For this review, take the finished solid that the model builds, in its own axes (mm). Face numbers are marked on the shaded views. A direction names the side the tool comes from. Coordinates: 2 decimals unless noted, no trailing zeros. Loops run counter-clockwise (first coordinate to the right, second up) from the corner with the lowest first, then second, coordinate; pieces in that order, holes last. Notation, with made-up numbers: (-14, 44.25) - (-1, 44.25) arc R9 ccw to (-1, 60.25) - close; hole circle Ø6 at (13, 78.25). An arc over 180 degrees is marked (long way). One line per item, written item: value. Start each with the question number.
1. Take a section at D-D, the plane z = -16.5. State the section outline as (x, y) points.
2. Take a section at B-B, the plane y = 4. State the section outline as (x, z) points, and give its area (3 significant figures).
3. For the marked faces 1, 2 and 3, list the 3-axis set-ups (+Z, -Z, +X, -X, +Y, -Y) from which the entire face can be reached by the end or side of a thin tool; tool diameter is ignored.
4. To check wall thickness, follow line 1 (Y direction, x = 25, z = 10.5); line 2 (X direction, y = 0.5, z = 0.5); line 3 (Z direction, x = 49.5, y = -8.5). State the ranges of each line that lie inside material, in increasing order. Write a range as from..to.
5. Take a section at C-C, the plane x = 43.5. State the section outline as (y, z) points, and give its area (3 significant figures).
6. Insertion check: pin 1 (8 mm diameter, centred on x = 46.5, z = -4, fed in from +Y); pin 2 (10 mm diameter, centred on x = 33, z = -12, fed in from -Y); pin 3 (10 mm diameter, centred on x = 18.5, y = -4.5, fed in from -Z); pin 4 (3 mm diameter, centred on y = 6.5, z = -9, fed in from +X). Each pin has a flat end and moves straight along its axis. Give the tip position at first contact, or say it passes through.
7. Take a section at A-A, the plane x = 51. State the section outline as (y, z) points.
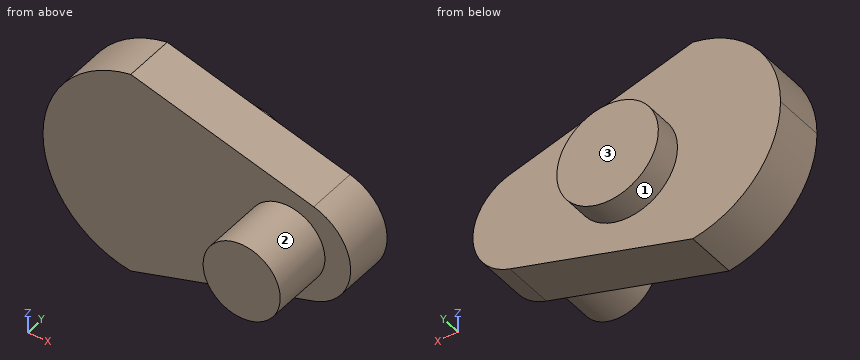
```python
from build123d import *

# Parameters (mm, degrees)
BOSS_EXTRUDE9_DEPTH  = 10
FILLET8_R            = 10
BOSS_EXTRUDE10_DEPTH = 5
SKETCH12_R           = 7.5
BOSS_EXTRUDE11_DEPTH = 12.5
SKETCH14_R           = 9.875
BOSS_EXTRUDE12_DEPTH = 0.25
CUT_EXTRUDE1_START   = -0.25
SKETCH15_R           = 7.5
CUT_EXTRUDE1_DEPTH   = 0.25
CUT_EXTRUDE2_START   = -12
SKETCH18_R           = 7.5
CUT_EXTRUDE2_DEPTH   = 12
SKETCH19_R           = 7.5
BOSS_EXTRUDE13_DEPTH = 12


with BuildPart() as part:
    # Sketch8 → Boss-Extrude9 (new body)
    with BuildSketch(Plane(origin=(0, 0, 0), x_dir=(1, 0, 0), z_dir=(0, 1, 0))):
        Polygon((17.063256467, 20), (17.063256467, 0), (85.43, 0), align=None)
        with BuildLine():
            ThreePointArc((17.063256467, 20), (4.845449314, 13.144910814), (0, 0))
            Line((0, 0), (17.063256467, 0))
            Line((17.063256467, 0), (17.063256467, 20))
        make_face()
        with BuildLine():
            Line((17.063256467, 0), (0, 0))
            ThreePointArc((0, 0), (4.845449314, -13.144910814), (17.063256467, -20))
            Line((17.063256467, -20), (17.063256467, 0))
        make_face()
        Polygon((85.43, 0), (17.063256467, 0), (17.063256467, -20), align=None)
    extrude(amount=BOSS_EXTRUDE9_DEPTH)

    # Fillet8
    fillet8_edges = [part.edges().sort_by_distance(p)[0] for p in [
        (85.43, 5, 0),
    ]]
    fillet(fillet8_edges, radius=FILLET8_R)

    # Sketch11 → Boss-Extrude10 (add)
    with BuildSketch(Plane(origin=(0, 10, 0), x_dir=(1, 0, 0), z_dir=(0, 1, 0))):
        with BuildLine():
            Line((20.031975788, 0), (29.906975788, 0))
            Line((29.906975788, 0), (39.781975788, 0))
            ThreePointArc((39.781975788, 0), (29.906975788, 9.875), (20.031975788, 0))
        make_face()
        with BuildLine():
            Line((39.781975788, 0), (29.906975788, 0))
            Line((29.906975788, 0), (20.031975788, 0))
            ThreePointArc((20.031975788, 0), (29.906975788, -9.875), (39.781975788, 0))
        make_face()
    extrude(amount=BOSS_EXTRUDE10_DEPTH)

    # Sketch12 → Boss-Extrude11 (add)
    with BuildSketch(Plane.XZ):
        with Locations(Location((47.313951576, 0, 0), (0, 0, 90))):
            Circle(SKETCH12_R)
    extrude(amount=BOSS_EXTRUDE11_DEPTH)

    # Sketch14 → Boss-Extrude12 (add)
    with BuildSketch(Plane(origin=(0, 15, 0), x_dir=(1, 0, 0), z_dir=(0, 1, 0))):
        with Locations(Location((29.906975788, 0, 0), (0, 0, 270))):
            Circle(SKETCH14_R)
    extrude(amount=BOSS_EXTRUDE12_DEPTH)

    # Sketch15 → Cut-Extrude1 (cut)
    with BuildSketch(Plane.XZ.offset(12.5).offset(CUT_EXTRUDE1_START)):
        with Locations(Location((47.313951576, 0, 0), (0, 0, 90))):
            Circle(SKETCH15_R)
    extrude(amount=CUT_EXTRUDE1_DEPTH, mode=Mode.SUBTRACT)

    # Sketch18 → Cut-Extrude2 (cut)
    with BuildSketch(Plane.XZ.offset(12.25).offset(CUT_EXTRUDE2_START)):
        with Locations(Location((47.313951576, 0, 0), (0, 0, 90))):
            Circle(SKETCH18_R)
    extrude(amount=CUT_EXTRUDE2_DEPTH, mode=Mode.SUBTRACT)

    # Sketch19 → Boss-Extrude13 (add)
    with BuildSketch(Plane.XZ.offset(0.25)):
        with Locations(Location((47.313951576, 0, 0), (0, 0, 90))):
            Circle(SKETCH19_R)
    extrude(amount=BOSS_EXTRUDE13_DEPTH)


solid = part.part
```
Solutions:
1. outline: (8.51, 0) - (29.03, 0) - (29.03, 10) - (8.51, 10) - close
2. outline: (17.06, -20) - (52.62, -9.6) arc R10 ccw to (52.62, 9.6) - (17.06, 20) arc R20.25 ccw to start
2. area: 1,670 mm2
3. face 1: +Y
3. face 2: -Y
3. face 3: +Z, -Z, +X, -X, +Y
4. line 1: 0..10
4. line 2: 0.01..59.8
4. line 3: -7.17..7.17
5. outline: (-12.25, -6.46) - (0, -6.46) - (0, -12.27) - (10, -12.27) - (10, 12.27) - (0, 12.27) - (0, 6.46) - (-12.25, 6.46) - close
5. area: 404 mm2
6. pin 1: y = 10
6. pin 2: y = 0
6. pin 3: z = -20
6. pin 4: x = 56.43
7. outline: (-12.25, -6.53) - (0, -6.53) - (0, -10.07) - (10, -10.07) - (10, 10.07) - (0, 10.07) - (0, 6.53) - (-12.25, 6.53) - close
